from build123d import *

# Parameters (mm, degrees)
SKETCH_W        = 32
SKETCH_H        = 20
PAD_DEPTH       = 60
SKETCH001_W     = 26
SKETCH001_H     = 5
POCKET_DEPTH    = 60.001
POCKET001_DEPTH = 60.001
SKETCH003_W     = 1.5
SKETCH003_H     = 6
POCKET002_DEPTH = 32.001


with BuildPart() as part:
    # Sketch → Pad (new body)
    with BuildSketch(Plane.XZ):
        with Locations((0, 10)):
            Rectangle(SKETCH_W, SKETCH_H)
    extrude(amount=PAD_DEPTH)

    # Sketch001 (on Face6 of Pad) → Pocket (cut, through all)
    with BuildSketch(Plane.XZ.offset(60)):
        with Locations((0, 17.5)):
            Rectangle(SKETCH001_W, SKETCH001_H)
    extrude(amount=-POCKET_DEPTH, mode=Mode.SUBTRACT)

    # Sketch002 (on Face5 of Pocket) → Pocket001 (cut, through all)
    with BuildSketch(Plane.XZ.offset(60)):
        with BuildLine():
            ThreePointArc((-2.000029, 12.5), (-10.838845, 8.838824), (-14.5, 0))
            Line((-14.5, 0), (14.5, 0))
            ThreePointArc((14.5, 0), (10.838845, 8.838824), (2.000029, 12.5))
            Line((-2.000029, 12.5), (2.000029, 12.5))
        make_face()
    extrude(amount=-POCKET001_DEPTH, mode=Mode.SUBTRACT)

    # Sketch003 (on Face9 of Pocket001) → Pocket002 (cut, through all)
    with BuildSketch(Plane(origin=(16, 0, 0), x_dir=(0, 0, 1), z_dir=(1, 0, 0))):
        with Locations((0.75, 55)):
            Rectangle(SKETCH003_W, SKETCH003_H)
        with Locations((0.75, 5)):
            Rectangle(SKETCH003_W, SKETCH003_H)
    extrude(amount=-POCKET002_DEPTH, mode=Mode.SUBTRACT)


solid = part.part
Can you work these out from the model? Positions are in its coordinate system, mm. A direction names the side the tool comes from. Coordinates: 2 decimals unless noted, no trailing zeros. Loops run counter-clockwise (first coordinate to the right, second up) from the corner with the lowest first, then second, coordinate; pieces in that order, holes last. Notation, with made-up numbers: M -18,6.25 L 29,6.25 A23 cw 29,29.25 Z; hole C -29,65 d8. An arc over 180 degrees is marked long. Return JSON: item names as keys, results as strings. Group by question number.
Item 1: Imagine slicing it at D-D (x = -6). Please give me the cut outline in (y, z), and give its area (3 significant figures).
Item 2: Imagine slicing it at A-A (z = 7.5). Please give me the cut outline in (x, y), and give its area (3 significant figures).
Item 3: Imagine slicing it at C-C (z = 17.5). Please give me the cut outline in (x, y).
Item 4: Thinking about a two-plate mould opening in Y: for faces 4 (the flat face through (-15, -2, 1)), 5 (the flat face through (-13, -30, 17)), 6 (the flat face through (0, -60, 13)), which applies, released by +Y, released by -Y, zero draft, split by the parting line, or undercut?
Item 5: On a 3-axis mill with a long thin cutter (end or side, diameter ignored), from which of +Z, -Z, +X, -X, +Y, -Y can I reach the whole of each face in a straight line? I mean faces 1 (the flat face through (0, -30, 12.5)), 2 (the flat face through (-15, -52, 1)), 3 (the flat face through (13, -30, 17)). Say none if no direction works.
Item 6: I'm going to push flat-ended pins straight in: pin 1 Ø1.2 at (x, z) = (-15, 1) entering from +Y; pin 2 Ø2 at (x, y) = (10, -14.5) entering from -Z; pin 3 Ø4 at (x, y) = (-11.5, -26.5) entering from -Z; pin 4 Ø1.2 at (x, y) = (1, -18.5) entering from -Z. Where does each tip first touch, or does it pass through?
Item 7: Imagine slicing it at B-B (y = -10). Please give me the cut outline in (x, z), and give its area (3 significant figures).
Item 8: If I drill on L1, parallel to X at y = -19, z = 19; L2, parallel to Z at x = -15, y = -53; L3, parallel to X at y = -17, z = 11.5, over which ranges is the centre line in solid material (lowest first)? Write a range as from..to.
Verdict:
{
 "1": {"outline": "M -60,11.84 L 0,11.84 L 0,15 L -60,15 Z", "area": "189 mm^2"},
 "2": {"outline": "M -16,-60 L -12,-60 L -12,0 L -16,0 Z; M 12,-60 L 16,-60 L 16,0 L 12,0 Z", "area": "480 mm^2"},
 "3": {"outline": "M -16,-60 L -13,-60 L -13,0 L -16,0 Z; M 13,-60 L 16,-60 L 16,0 L 13,0 Z"},
 "4": {"face 4": "undercut", "face 5": "zero draft", "face 6": "released by -Y"},
 "5": {"face 1": "-Z, +Y, -Y", "face 2": "-Z, +X, -X", "face 3": "+Z, +Y, -Y"},
 "6": {"pin 1": "stops at y = 0", "pin 2": "stops at z = 8.67", "pin 3": "stops at z = 4.9", "pin 4": "stops at z = 12.5"},
 "7": {"outline": "M -16,0 L -14.5,0 A12.5 cw -2,12.5 L 2,12.5 A12.5 cw 14.5,0 L 16,0 L 16,20 L 13,20 L 13,15 L -13,15 L -13,20 L -16,20 Z", "area": "215 mm^2"},
 "8": {"L1": "x = -16..-13, 13..16", "L2": "z = 1.5..20", "L3": "x = -16..-6.9, 6.9..16"}
}
